The model under review builds one solid part; all positions refer to its coordinate system, in mm. Face numbers are marked on the shaded views. A direction names the side the tool comes from. Coordinates: 2 decimals unless noted, no trailing zeros. Loops run counter-clockwise (first coordinate to the right, second up) from the corner with the lowest first, then second, coordinate; pieces in that order, holes last. Notation, with made-up numbers: M 9,35.25 L 64,35.25 A37 ccw 64,72.25 Z; hole C 62.5,17 d5. An arc over 180 degrees is marked long. Use one line per item in the form item = value.
```python
from build123d import *

# Parameters (mm, degrees)
EXTRUDE_1_DEPTH     = 30
SKETCH_4_R          = 1.5
CUT_EXTRUDE_3_DEPTH = 2
SKETCH_5_R          = 13.5
CUT_EXTRUDE_4_DEPTH = 5


with BuildPart() as part:
    # 草图1 → 凸台-拉伸1 (new body)
    with BuildSketch(Plane.XY):
        Polygon((-21.167340442, 37.672826145), (-21.167340442, 27.672826145), (-2.167340442, 27.672826145), (-2.167340442, 58.672826145), (15.832659558, 58.672826145), (15.832659558, 57.672826145), (-1.167340442, 57.672826145), (-1.167340442, 26.672826145), (-22.167340442, 26.672826145), (-22.167340442, 37.672826145), align=None)
    extrude(amount=EXTRUDE_1_DEPTH)

    # 草图4 → 切除-拉伸3 (cut)
    with BuildSketch(Plane.ZY.offset(22.167340442)):
        with Locations((15, 30.972826145)):
            Circle(SKETCH_4_R)
    extrude(amount=-CUT_EXTRUDE_3_DEPTH, mode=Mode.SUBTRACT)

    # 草图5 → 切除-拉伸4 (cut)
    with BuildSketch(Plane.ZY.offset(2.167340442)):
        with Locations((15, 43.172826145)):
            Circle(SKETCH_5_R)
    extrude(amount=-CUT_EXTRUDE_4_DEPTH, mode=Mode.SUBTRACT)


solid = part.part
```
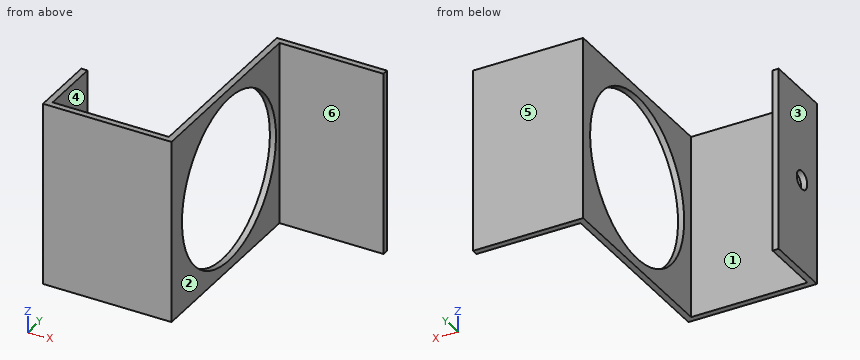
1. Add section D-D (x = 11). State the section outline as (y, z) points, then the cut area to 3 significant figures.
Response values:
outline = M 57.67,0 L 58.67,0 L 58.67,30 L 57.67,30 Z
area = 30.0 mm^2
2. Add section C-C (z = 15). State the section outline as (x, y) points, then the cut area to 3 significant figures.
Response values:
outline = M -22.17,26.67 L -1.17,26.67 L -1.17,29.67 L -2.17,29.67 L -2.17,27.67 L -21.17,27.67 L -21.17,29.47 L -22.17,29.47 Z; M -22.17,32.47 L -21.17,32.47 L -21.17,37.67 L -22.17,37.67 Z; M -2.17,56.67 L -1.17,56.67 L -1.17,57.67 L 15.83,57.67 L 15.83,58.67 L -2.17,58.67 Z
area = 49.0 mm^2
3. Insertion check: P1, Ø3, axis at y = 31, z = 24, coming from the +X side; P2, Ø1.1, axis at x = -21.5, z = 12, coming from the +Y side. Each pin has a flat end and moves straight along its axis. Give the tip position at first contact, or say it passes through.
Response values:
P1 = -1.17
P2 = 37.67
4. Wall thickness on line 1 along X through (y, z) = (30, 25.5); line 2 along Y through (x, z) = (-21.9, 15); line 3 along X through (y, z) = (36, 7): over which ranges is each line inside the solid? List them lowest first. Write a range as from..to.
Response values:
line_1 = -22.17..-21.17, -2.17..-1.17
line_2 = 26.67..29.47, 32.47..37.67
line_3 = -22.17..-21.17
5. Add section B-B (y = 47). State the section outline as (x, z) points.
Response values:
outline = M -2.17,0 L -1.17,0 L -1.17,2.05 L -2.17,2.05 Z; M -2.17,27.95 L -1.17,27.95 L -1.17,30 L -2.17,30 Z
6. The part is to be moulded in two halves that separate along X. For the marked faces 1, 2 and 3, say which applies: pulls with the +X half, pulls with the -X half, needs draft (parallel to the pull), parting line crosses it, or undercut.
Response values:
face_1 = undercut
face_2 = pulls with the +X half
face_3 = pulls with the -X half
7. Add section A-A (z = 27.5). State the section outline as (x, y) points.
Response values:
outline = M -22.17,26.67 L -1.17,26.67 L -1.17,38.07 L -2.17,38.07 L -2.17,27.67 L -21.17,27.67 L -21.17,37.67 L -22.17,37.67 Z; M -2.17,48.27 L -1.17,48.27 L -1.17,57.67 L 15.83,57.67 L 15.83,58.67 L -2.17,58.67 Z
8. Machinability: for the marked faces 4, 5 and 6, which of the approach directions +Z, -Z, +X, -X, +Y, -Y give a long, thin tool a straight path to every point of the face, cutting with its end or side? Answer none if there is none.
Response values:
face_4 = +Z, -Z, +Y
face_5 = +Z, -Z, +X, -X, +Y
face_6 = +Z, -Z, +X, -Y
